Check sheet for the modelled part. Datum: model origin and axes. Units: mm. Face numbers are marked on the shaded views. A direction names the side the tool comes from. Coordinates: 2 decimals unless noted, no trailing zeros. Loops run counter-clockwise (first coordinate to the right, second up) from the corner with the lowest first, then second, coordinate; pieces in that order, holes last. Notation, with made-up numbers: M -15,73.25 L 35,73.25 A32 ccw 35,104.25 Z; hole C 78,21 d6. An arc over 180 degrees is marked long. Answer as CSV lines item,"result". Start each with the question number.
from build123d import *

# Parameters (mm, degrees)
SKETCH1_R           = 25
BOSS_EXTRUDE2_DEPTH = 2.5
SCALE1_SCALE        = 1.5


with BuildPart() as part:
    # Sketch1 → Boss-Extrude2 (new, symmetric)
    with BuildSketch(Plane.XY):
        Circle(SKETCH1_R)
        with BuildLine():
            Line((0, 22.5), (-3.040407483, 17.233859763))
            ThreePointArc((-3.040407483, 17.233859763), (-1.526016734, 17.433337974), (0, 17.5))
            Line((0, 17.5), (2.786730187, 22.32675827))
            ThreePointArc((2.786730187, 22.32675827), (8.267212977, 20.926136519), (13.225168177, 18.202882373))
            Line((13.225168177, 18.202882373), (7.670067285, 15.729592107))
            ThreePointArc((7.670067285, 15.729592107), (9.012485488, 15.000836821), (10.286241915, 14.157797402))
            Line((10.286241915, 14.157797402), (15.377851323, 16.424727964))
            ThreePointArc((15.377851323, 16.424727964), (18.988390227, 12.070254205), (21.398771617, 6.952882373))
            Line((21.398771617, 6.952882373), (15.450837046, 8.217154895))
            ThreePointArc((15.450837046, 8.217154895), (16.108524577, 6.838525862), (16.643489035, 5.407797402))
            Line((16.643489035, 5.407797402), (22.095155927, 4.249009832))
            ThreePointArc((22.095155927, 4.249009832), (22.456647803, -1.396054962), (21.398771617, -6.952882373))
            Line((21.398771617, -6.952882373), (17.329912211, -2.433956196))
            ThreePointArc((17.329912211, -2.433956196), (17.051654786, -3.935869544), (16.643489035, -5.407797402))
            Line((16.643489035, -5.407797402), (20.372861954, -9.549685638))
            ThreePointArc((20.372861954, -9.549685638), (17.347229191, -14.329118584), (13.225168177, -18.202882373))
            Line((13.225168177, -18.202882373), (12.589549933, -12.155378747))
            ThreePointArc((12.589549933, -12.155378747), (11.481632431, -13.206896559), (10.286241915, -14.157797402))
            Line((10.286241915, -14.157797402), (10.868827163, -19.700725776))
            ThreePointArc((10.868827163, -19.700725776), (5.611758639, -21.788945935), (0, -22.5))
            Line((0, -22.5), (3.040407483, -17.233859763))
            ThreePointArc((3.040407483, -17.233859763), (1.526016734, -17.433337974), (0, -17.5))
            Line((0, -17.5), (-2.786730187, -22.32675827))
            ThreePointArc((-2.786730187, -22.32675827), (-8.267212977, -20.926136519), (-13.225168177, -18.202882373))
            Line((-13.225168177, -18.202882373), (-7.670067285, -15.729592107))
            ThreePointArc((-7.670067285, -15.729592107), (-9.012485488, -15.000836821), (-10.286241915, -14.157797402))
            Line((-10.286241915, -14.157797402), (-15.377851323, -16.424727964))
            ThreePointArc((-15.377851323, -16.424727964), (-18.988390227, -12.070254205), (-21.398771617, -6.952882373))
            Line((-21.398771617, -6.952882373), (-15.450837046, -8.217154895))
            ThreePointArc((-15.450837046, -8.217154895), (-16.108524577, -6.838525862), (-16.643489035, -5.407797402))
            Line((-16.643489035, -5.407797402), (-22.095155927, -4.249009832))
            ThreePointArc((-22.095155927, -4.249009832), (-22.456647803, 1.396054962), (-21.398771617, 6.952882373))
            Line((-21.398771617, 6.952882373), (-17.329912211, 2.433956196))
            ThreePointArc((-17.329912211, 2.433956196), (-17.051654786, 3.935869544), (-16.643489035, 5.407797402))
            Line((-16.643489035, 5.407797402), (-20.372861954, 9.549685638))
            ThreePointArc((-20.372861954, 9.549685638), (-17.347229191, 14.329118584), (-13.225168177, 18.202882373))
            Line((-13.225168177, 18.202882373), (-12.589549933, 12.155378747))
            ThreePointArc((-12.589549933, 12.155378747), (-11.481632431, 13.206896559), (-10.286241915, 14.157797402))
            Line((-10.286241915, 14.157797402), (-10.868827163, 19.700725776))
            ThreePointArc((-10.868827163, 19.700725776), (-5.611758639, 21.788945935), (0, 22.5))
        make_face(mode=Mode.SUBTRACT)
    extrude(amount=BOSS_EXTRUDE2_DEPTH, both=True)


with BuildPart() as part_1:
    # Scale1: scaled about (0, 0, 0)
    add(part.part.scale(SCALE1_SCALE))


solid = part_1.part
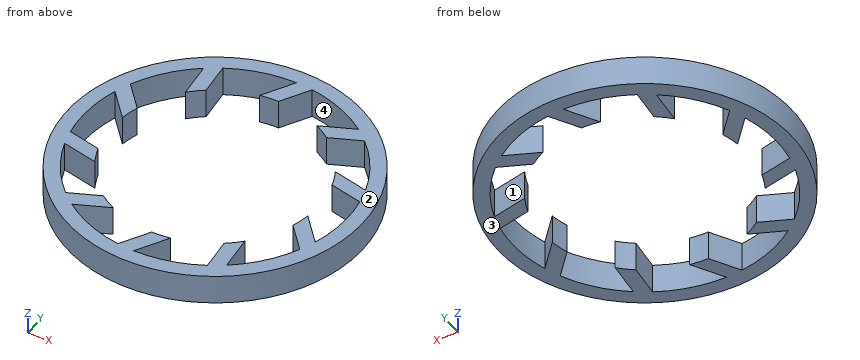
Item 1: Sectioned sample at C-C, the plane x = 12.5. Record the boundary of the cut face in (y, z).
Item 2: Sectioned sample at D-D, the plane x = 28.5. Record the boundary of the cut face in (y, z), and give its area (3 significant figures).
Item 3: Set-up check for the marked faces 1 and 2: record each of +Z, -Z, +X, -X, +Y, -Y from which the full face is reachable in a straight line by a thin tool's end or side.
Item 4: Material ranges on line 1 (X direction, y = 19, z = 2.5); line 2 (X direction, y = -24, z = -1.5); line 3 (Y direction, x = -12, z = -2.5), recorded low to high. Write a range as from..to.
Item 5: Go/stop test with flat-tipped pins: pin 1 (8 mm diameter, centred on x = -26, y = 12, fed in from -Z); pin 2 (4 mm diameter, centred on x = -19.5, z = 1.5, fed in from +Y); pin 3 (1.5 mm diameter, centred on x = 21.5, z = 1.5, fed in from +Y); pin 4 (1 mm diameter, centred on x = 23, z = -2.5, fed in from +Y). Record where each tip stops, or that it passes through.
Item 6: Sectioned sample at B-B, the plane y = -31. Record the boundary of the cut face in (x, z).
Item 7: Sectioned sample at A-A, the plane y = 0. Record the boundary of the cut face in (x, z).
Item 8: Release check for a two-part mould opening along X. For the marked faces 3 and 4 record: released by +X, released by -X, zero draft, split by the parting line, or undercut.
Reply:
1,outline,"M -35.36,-3.75 L -31.35,-3.75 L -31.35,3.75 L -35.36,3.75 Z; M 23.08,-3.75 L 24.04,-3.75 L 24.04,3.75 L 23.08,3.75 Z; M 31.35,-3.75 L 35.36,-3.75 L 35.36,3.75 L 31.35,3.75 Z"
2,outline,"M -24.37,-3.75 L -18.08,-3.75 L -18.08,3.75 L -24.37,3.75 Z; M -12.04,-3.75 L -6.43,-3.75 L -6.43,3.75 L -12.04,3.75 Z; M 7.36,-3.75 L 11.19,-3.75 L 11.19,3.75 L 7.36,3.75 Z; M 18.08,-3.75 L 24.37,-3.75 L 24.37,3.75 L 18.08,3.75 Z"
2,area,"165 mm²"
3,face 1,"+Z, -Z"
3,face 2,"+Z, +X, -X, +Y, -Y"
4,line 1,"-32.33..-27.89, -18.96..-18.11, 27.89..32.33"
4,line 2,"-28.81..-23.73, -21.64..-12.42, 15.72..19.49, 23.73..28.81"
4,line 3,"-35.53..-31.54, -23.81..-23.35, 31.54..35.53"
5,pin 1,"z = -3.75"
5,pin 2,"y = 33.17"
5,pin 3,"y = 31.24"
5,pin 4,"y = 30"
6,outline,"M -21.1,-3.75 L -13.34,-3.75 L -13.34,3.75 L -21.1,3.75 Z; M -2.74,-3.75 L 1.59,-3.75 L 1.59,3.75 L -2.74,3.75 Z; M 13.34,-3.75 L 21.1,-3.75 L 21.1,3.75 L 13.34,3.75 Z"
7,outline,"M -37.5,-3.75 L -33.75,-3.75 L -33.75,3.75 L -37.5,3.75 Z; M 33.75,-3.75 L 37.5,-3.75 L 37.5,3.75 L 33.75,3.75 Z"
8,face 3,"zero draft"
8,face 4,"undercut"
